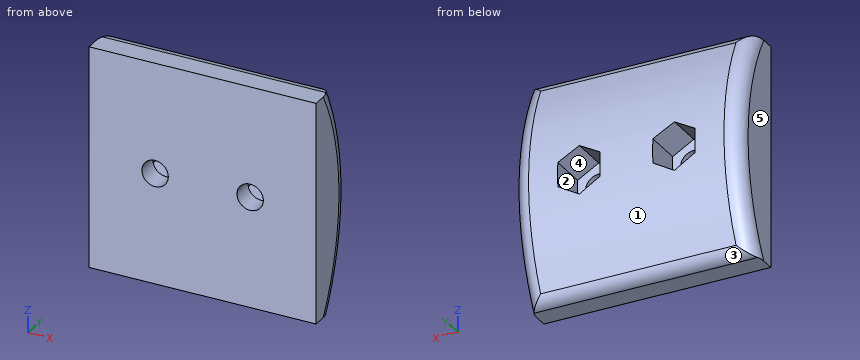
```python
from build123d import *

# Parameters (mm, degrees)
BOSS_EXTRUDE1_DEPTH = 21.5
FILLET1_R           = 3
CUT_EXTRUDE1_START  = -4
CUT_EXTRUDE1_DEPTH  = 29.073373183
SKETCH4_R           = 2.5
CUT_EXTRUDE2_DEPTH  = 4


with BuildPart() as part:
    # Sketch2 → Boss-Extrude1 (new, symmetric)
    with BuildSketch(Plane(origin=(0, 0, 0), x_dir=(0, 0, -1), z_dir=(1, 0, 0))):
        with BuildLine():
            Line((-21, 6), (-21, 0))
            Line((-21, 0), (21, 0))
            Line((21, 0), (21, 6))
            ThreePointArc((21, 6), (0, 11.200502516), (-21, 6))
        make_face()
    extrude(amount=BOSS_EXTRUDE1_DEPTH, both=True)

    # Fillet1
    fillet1_edges = [part.edges().sort_by_distance(p)[0] for p in [
        (21.5, 11.200502516, 0),
        (-21.5, 11.200502516, 0),
        (0, 6, -21),
        (0, 6, 21),
    ]]
    fillet(fillet1_edges, radius=FILLET1_R)

    # Sketch3 → Cut-Extrude1 (cut, through all)
    with BuildSketch(Plane.XZ.offset(CUT_EXTRUDE1_START)):
        Polygon((5, 2.309401077), (5, -2.309401077), (9, -4.618802154), (13, -2.309401077), (13, 2.309401077), (9, 4.618802154), align=None)
        Polygon((-9, 4.618802154), (-5, 2.309401077), (-5, -2.309401077), (-9, -4.618802154), (-13, -2.309401077), (-13, 2.309401077), align=None)
    extrude(amount=-CUT_EXTRUDE1_DEPTH, mode=Mode.SUBTRACT)

    # Sketch4 → Cut-Extrude2 (cut)
    with BuildSketch(Plane.XZ):
        with Locations(Location((9, 0, 0), (0, 0, 270))):
            Circle(SKETCH4_R)
        with Locations(Location((-9, 0, 0), (0, 0, 270))):
            Circle(SKETCH4_R)
    extrude(amount=-CUT_EXTRUDE2_DEPTH, mode=Mode.SUBTRACT)


solid = part.part
```
Can you work these out from the model? Positions are in its coordinate system, mm. Face numbers are marked on the shaded views. A direction names the side the tool comes from. Round coordinates to 2 decimals unless told otherwise and drop trailing zeros. Loops run counter-clockwise (first coordinate to the right, second up) from the corner with the lowest first, then second, coordinate; pieces in that order, holes last. Notation, with made-up numbers: (-39, -6) -> (19, -6) arc R14 cw to (19, 7) -> close; hole circle Ø1 at (77, -8.75). An arc over 180 degrees is marked (long way). One line per item, written item: value. Start each with the question number.
1. If we section it at C-C, the plane x = -12: Write out the boundary of the cut face in (y, z), then the cut area to 3 significant figures.
2. If we section it at B-B, the plane x = 10.5: Write out the boundary of the cut face in (y, z).
3. If I drill on probe 1 along X at (y, z) = (1.2, 0); probe 2 along X at (y, z) = (7.25, -0.5); probe 3 along Y at (x, z) = (2.5, -1), over which ranges is the centre line in solid material (lowest first)?
4. For the marked faces 4 and 5, which set-ups out of +Z, -Z, +X, -X, +Y, -Y let a thin tool reach every point of the face, with its end or its side?
5. If we mould it in two halves opening along Z, with no side actions, what happens to the marked faces 1, 2 and 3? For each: pulls with the +Z half, pulls with the -Z half, needs draft (parallel to the pull), parting line crosses it, or undercut.
6. If we section it at A-A, the plane z = 0: Write out the boundary of the cut face in (x, y), then the cut area to 3 significant figures.
7. If we section it at D-D, the plane y = 9.25: Give the number of separate pieces and of enclosed holes in the cut face, then the cut area to 3 significant figures.
8. For pin 1 (1 mm diameter, centred on x = 13.5, z = -2, fed in from +Y), with a flat end and sliding along its axis, tell me the tip position at first contact or that it passes through.
Calculated:
1. outline: (0, -21) -> (4.15, -21) arc R3 ccw to (6.86, -19.29) arc R45 ccw to (11.11, -2.89) -> (4, -2.89) -> (4, 2.89) -> (11.11, 2.89) arc R45 ccw to (6.86, 19.29) arc R3 ccw to (4.15, 21) -> (0, 21) -> close
1. area: 357 mm²
2. outline: (0, -21) -> (4.15, -21) arc R3 ccw to (6.86, -19.29) arc R45 ccw to (11.04, -3.75) -> (4, -3.75) -> (4, -2) -> (0, -2) -> close; (0, 2) -> (4, 2) -> (4, 3.75) -> (11.04, 3.75) arc R45 ccw to (6.86, 19.29) arc R3 ccw to (4.15, 21) -> (0, 21) -> close
3. probe 1: x = -21.5 to -11.5, -6.5 to 6.5, 11.5 to 21.5
3. probe 2: x = -21.5 to -13, -5 to 5, 13 to 21.5
3. probe 3: y = 0 to 11.19
4. face 4: +Y
4. face 5: +Z, -Z, -X, +Y, -Y
5. face 1: parting line crosses it
5. face 2: undercut
5. face 3: pulls with the -Z half
6. outline: (-21.5, 0) -> (-11.5, 0) -> (-11.5, 4) -> (-13, 4) -> (-13, 11.2) -> (-18.5, 11.2) arc R3 ccw to (-21.5, 8.2) -> close; (-6.5, 0) -> (6.5, 0) -> (6.5, 4) -> (5, 4) -> (5, 11.2) -> (-5, 11.2) -> (-5, 4) -> (-6.5, 4) -> close; (11.5, 0) -> (21.5, 0) -> (21.5, 8.2) arc R3 ccw to (18.5, 11.2) -> (13, 11.2) -> (13, 4) -> (11.5, 4) -> close
6. area: 323 mm²
7. separate pieces: 1
7. enclosed holes: 2
7. area: 981 mm²
8. pin 1: stops at y = 11.18
